```python
from build123d import *

# Parameters (mm, degrees)
F1_DEPTH  = 4.445
F3_DEPTH  = 1.778
F5_R      = 38.1
F6_DEPTH  = 31.75
F4_R      = 34.925
F7_DEPTH  = 28.575
F10_DEPTH = 25.4
F11_DEPTH = 22.225
F12_R     = 1.5875
F13_W     = 1.778
F13_H     = 20.066
F14_DEPTH = 2.54
F15_W     = 1.778
F15_H     = 20.066
F16_DEPTH = 2.54
F17_W     = 1.778
F17_H     = 20.066
F18_DEPTH = 2.54
F19_W     = 1.778
F19_H     = 20.066
F20_DEPTH = 2.54
F22_DEPTH = 2.54
F23_START = -86.2838
F23_DEPTH = 2.54


with BuildPart() as f1:
    # F0 (on Front) → F1 (new body)
    with BuildSketch(Plane.XZ):
        with BuildLine():
            Line((40.6019, 72.8091), (-40.6019, 72.8091))
            ThreePointArc((-40.6019, 72.8091), (-43.2959768363, 71.6931768363), (-44.4119, 68.9991))
            Line((-44.4119, 68.9991), (-44.4119, -68.9991))
            ThreePointArc((-44.4119, -68.9991), (-43.2959768363, -71.6931768363), (-40.6019, -72.8091))
            Line((-40.6019, -72.8091), (40.6019, -72.8091))
            ThreePointArc((40.6019, -72.8091), (43.2959768363, -71.6931768363), (44.4119, -68.9991))
            Line((44.4119, -68.9991), (44.4119, 68.9991))
            ThreePointArc((44.4119, 68.9991), (43.2959768363, 71.6931768363), (40.6019, 72.8091))
        make_face()
    extrude(amount=F1_DEPTH)

    # F2 (on face) → F3 (cut)
    with BuildSketch(Plane.XZ):
        with BuildLine():
            Line((41.8719, -67.7291), (41.8719, 67.7291))
            ThreePointArc((41.8719, 67.7291), (41.1279512242, 69.5251512242), (39.3319, 70.2691))
            Line((39.3319, 70.2691), (-39.3319, 70.2691))
            ThreePointArc((-39.3319, 70.2691), (-41.1279512242, 69.5251512242), (-41.8719, 67.7291))
            Line((-41.8719, 67.7291), (-41.8719, -67.7291))
            ThreePointArc((-41.8719, -67.7291), (-41.1279512242, -69.5251512242), (-39.3319, -70.2691))
            Line((-39.3319, -70.2691), (39.3319, -70.2691))
            ThreePointArc((39.3319, -70.2691), (41.1279512242, -69.5251512242), (41.8719, -67.7291))
        make_face()
    extrude(amount=F3_DEPTH, mode=Mode.SUBTRACT)

    # F5 (on face) → F6 (join)
    with BuildSketch(Plane.XZ.offset(4.445)):
        with Locations((0, 28.3591)):
            Circle(F5_R)
    extrude(amount=-F6_DEPTH)

    # F4 (on face) → F7 (cut)
    with BuildSketch(Plane.XZ.offset(4.445)):
        with Locations((0, 28.3591)):
            Circle(F4_R)
    extrude(amount=-F7_DEPTH, mode=Mode.SUBTRACT)

    # F8 (on face) → F10 (join)
    with BuildSketch(Plane.XZ.offset(4.445)):
        with BuildLine():
            Line((35.5219, -16.9291), (-35.5219, -16.9291))
            ThreePointArc((-35.5219, -16.9291), (-37.3179512242, -17.6730487758), (-38.0619, -19.4691))
            Line((-38.0619, -19.4691), (-38.0619, -63.9191))
            ThreePointArc((-38.0619, -63.9191), (-37.3179512242, -65.7151512242), (-35.5219, -66.4591))
            Line((-35.5219, -66.4591), (35.5219, -66.4591))
            ThreePointArc((35.5219, -66.4591), (37.3179512242, -65.7151512242), (38.0619, -63.9191))
            Line((38.0619, -63.9191), (38.0619, -19.4691))
            ThreePointArc((38.0619, -19.4691), (37.3179512242, -17.6730487758), (35.5219, -16.9291))
        make_face()
    extrude(amount=-F10_DEPTH)

    # F9 (on face) → F11 (cut)
    with BuildSketch(Plane.XZ.offset(4.445)):
        with BuildLine():
            Line((32.9819, -20.1041), (-32.9819, -20.1041))
            ThreePointArc((-32.9819, -20.1041), (-34.3289384182, -20.6620615818), (-34.8869, -22.0091))
            Line((-34.8869, -22.0091), (-34.8869, -61.3791))
            ThreePointArc((-34.8869, -61.3791), (-34.3289384182, -62.7261384182), (-32.9819, -63.2841))
            Line((-32.9819, -63.2841), (32.9819, -63.2841))
            ThreePointArc((32.9819, -63.2841), (34.3289384182, -62.7261384182), (34.8869, -61.3791))
            Line((34.8869, -61.3791), (34.8869, -22.0091))
            ThreePointArc((34.8869, -22.0091), (34.3289384182, -20.6620615818), (32.9819, -20.1041))
        make_face()
    extrude(amount=-F11_DEPTH, mode=Mode.SUBTRACT)

    # F12
    f12_edges = [f1.edges().sort_by_distance(p)[0] for p in [
        (34.8869, 17.78, -41.6941),
        (34.328938, 17.78, -20.662062),
        (0, 17.78, -20.1041),
        (-34.328938, 17.78, -20.662062),
        (-34.8869, 17.78, -41.6941),
        (-34.328938, 17.78, -62.726138),
        (0, 17.78, -63.2841),
        (34.328938, 17.78, -62.726138),
        (-34.925, 24.13, 28.3591),
    ]]
    fillet(f12_edges, radius=F12_R)

    # F13 (on face) → F14 (cut)
    with BuildSketch(Plane.YZ.offset(44.4119)):
        with Locations((-0.889, -44.9961)):
            Rectangle(F13_W, F13_H)
    extrude(amount=-F14_DEPTH, mode=Mode.SUBTRACT)

    # F15 (on face) → F16 (cut)
    with BuildSketch(Plane(origin=(-44.4119, 0, 0), x_dir=(0, -1, 0), z_dir=(-1, 0, 0))):
        with Locations((0.889, -44.9961)):
            Rectangle(F15_W, F15_H)
    extrude(amount=-F16_DEPTH, mode=Mode.SUBTRACT)

    # F17 (on face) → F18 (cut)
    with BuildSketch(Plane.YZ.offset(44.4119)):
        with Locations((-0.889, 47.5361)):
            Rectangle(F17_W, F17_H)
    extrude(amount=-F18_DEPTH, mode=Mode.SUBTRACT)

    # F19 (on face) → F20 (cut)
    with BuildSketch(Plane(origin=(-44.4119, 0, 0), x_dir=(0, -1, 0), z_dir=(-1, 0, 0))):
        with Locations((0.889, 47.5361)):
            Rectangle(F19_W, F19_H)
    extrude(amount=-F20_DEPTH, mode=Mode.SUBTRACT)

    # F21 (on face) → F22 (join)
    with BuildSketch(Plane.YZ.offset(44.4119)):
        Polygon((-1.778, -46.1137), (-1.778, -49.1871), (3.302, -49.1871), (4.318, -51.6636), (6.858, -51.6636), (10.922, -49.1871), (10.922, -48.1711), (3.3188345842, -46.1137), align=None)
        Polygon((-1.778, -40.8051), (-1.778, -43.8785), (3.3188345842, -43.8785), (10.922, -41.8211), (10.922, -40.8051), (6.858, -38.3286), (4.318, -38.3286), (3.302, -40.8051), align=None)
        Polygon((-1.778, 46.4185), (-1.778, 43.3451), (3.302, 43.3451), (4.318, 40.8686), (6.858, 40.8686), (10.922, 43.3451), (10.922, 44.3611), (3.3188345842, 46.4185), align=None)
        Polygon((3.302, 51.7271), (-1.778, 51.7271), (-1.778, 48.6537), (3.3188345842, 48.6537), (10.922, 50.7111), (10.922, 51.7271), (6.858, 54.2036), (4.318, 54.2036), align=None)
    extrude(amount=-F22_DEPTH)

    # F21 (on face) → F23 (join)
    with BuildSketch(Plane.YZ.offset(44.4119).offset(F23_START)):
        Polygon((-1.778, -46.1137), (-1.778, -49.1871), (3.302, -49.1871), (4.318, -51.6636), (6.858, -51.6636), (10.922, -49.1871), (10.922, -48.1711), (3.3188345842, -46.1137), align=None)
        Polygon((-1.778, -40.8051), (-1.778, -43.8785), (3.3188345842, -43.8785), (10.922, -41.8211), (10.922, -40.8051), (6.858, -38.3286), (4.318, -38.3286), (3.302, -40.8051), align=None)
        Polygon((-1.778, 46.4185), (-1.778, 43.3451), (3.302, 43.3451), (4.318, 40.8686), (6.858, 40.8686), (10.922, 43.3451), (10.922, 44.3611), (3.3188345842, 46.4185), align=None)
        Polygon((3.302, 51.7271), (-1.778, 51.7271), (-1.778, 48.6537), (3.3188345842, 48.6537), (10.922, 50.7111), (10.922, 51.7271), (6.858, 54.2036), (4.318, 54.2036), align=None)
    extrude(amount=-F23_DEPTH)


solid = f1.part
```
Model file for the job. Use its own axes, mm. A direction names the side the tool comes from. Coordinates: 2 decimals unless noted, no trailing zeros. Write each loop counter-clockwise with the first axis right and the second up, starting at its lowest first coordinate (ties: lowest second). Pieces come first, ordered by that corner, then holes. Notation, with made-up numbers: (66, 75) - (94, 75) arc R28 ccw to (94, 96) - close; hole circle Ø8 at (-40, 34). An arc over 180 degrees is marked (long way). Use a Markdown table: item, result. Add a question column.
Item 1: Band-saw the part on C-C, the plane y = 9. Give the number of separate pieces and of enclosed holes in the cut face, and give its area (3 significant figures).
Item 2: 3-axis set-ups, long thin cutter, end or side, ignore diameter. For faces 1 (the face through (-1, 20.955, -41)), 2 (the face through (-8.259, 12.56, -8.835)), 3 (the face through (0, 6, -63.284)): which of +Z, -Z, +X, -X, +Y, -Y reach the whole face in a straight line?
Item 3: Band-saw the part on A-A, the plane x = 0. Write the cut outline in (y, z) (1 decimal), and give its area (3 significant figures).
Item 4: Drill centre lines: line 1 along Z through (x, y) = (0, 2.25); line 2 along X through (y, z) = (10, -25.5); line 3 along Z through (x, y) = (8.5, -3). Where is each one in solid material? Low to high.
Item 5: Band-saw the part on B-B, the plane z = -56.5. Write the cut outline in (x, y) (1 decimal), and give its area (3 significant figures).
Item 6: Drop flat-ended pins along their axis: pin 1 (1.4 mm diameter, centred on x = 43, y = -0.5, fed in from +Z); pin 2 (3 mm diameter, centred on y = 7, z = -1.5, fed in from +X); pin 3 (1.5 mm diameter, centred on x = -6.5, y = 16.5, fed in from -Z). Give the stop position or say it passes through.
Item 7: Two-plate mould, pull along Z, no slides. Class faces 4 (the face through (0, 24.13, 29)), 5 (the face through (-43.27, -2.19, 71.72)), 6 (the face through (44.412, -2, -1)): pulls with the +Z half, pulls with the -Z half, needs draft (parallel to the pull), parting line crosses it, or undercut.
A:
| question | item | result |
|---|---|---|
| 1 | separate pieces | 10 |
| 1 | enclosed holes | 2 |
| 1 | area | 1,540 mm² |
| 2 | face 1 | -Z, +X, -X, +Y |
| 2 | face 2 | +Y |
| 2 | face 3 | -Y |
| 3 | outline | (-4.4, -72.8) - (0, -72.8) - (0, -70.3) - (-1.8, -70.3) - (-1.8, -66.5) - (21, -66.5) - (21, -16.9) - (-1.8, -16.9) - (-1.8, -9.7) - (27.3, -9.7) - (27.3, 66.5) - (-1.8, 66.5) - (-1.8, 70.3) - (0, 70.3) - (0, 72.8) - (-4.4, 72.8) - (-4.4, 63.3) - (22.5, 63.3) arc R1.6 cw to (24.1, 61.7) - (24.1, -5) arc R1.6 cw to (22.5, -6.6) - (-4.4, -6.6) - (-4.4, -20.1) - (16.2, -20.1) arc R1.6 cw to (17.8, -21.7) - (17.8, -61.7) arc R1.6 cw to (16.2, -63.3) - (-4.4, -63.3) - close |
| 3 | area | 786 mm² |
| 4 | line 1 | z = -66.46 to -63.28, -20.1 to -16.93, -9.74 to -6.57, 63.28 to 66.46 |
| 4 | line 2 | x = -38.06 to -34.89, 34.89 to 38.06 |
| 4 | line 3 | z = -72.81 to -63.28, -20.1 to -5.52, 62.23 to 72.81 |
| 5 | outline | (-44.4, -4.4) - (-34.9, -4.4) - (-34.9, 16.2) arc R1.6 cw to (-33.3, 17.8) - (33.3, 17.8) arc R1.6 cw to (34.9, 16.2) - (34.9, -4.4) - (44.4, -4.4) - (44.4, 0) - (41.9, 0) - (41.9, -1.8) - (38.1, -1.8) - (38.1, 21) - (-38.1, 21) - (-38.1, -1.8) - (-41.9, -1.8) - (-41.9, 0) - (-44.4, 0) - close |
| 5 | area | 427 mm² |
| 6 | pin 1 | stops at z = 72.41 |
| 6 | pin 2 | stops at x = 25.44 |
| 6 | pin 3 | stops at z = -66.46 |
| 7 | face 4 | undercut |
| 7 | face 5 | pulls with the +Z half |
| 7 | face 6 | needs draft |
